The model under review builds one solid part; all positions refer to its coordinate system, in mm. A direction names the side the tool comes from. Coordinates: 2 decimals unless noted, no trailing zeros. Write each loop counter-clockwise with the first axis right and the second up, starting at its lowest first coordinate (ties: lowest second). Pieces come first, ordered by that corner, then holes. Notation, with made-up numbers: (74, 53.25) - (82, 53.25) arc R14 cw to (82, 72.25) - close; hole circle Ø10 at (41.25, 32.25). An arc over 180 degrees is marked (long way). Use one line per item in the form item = value. Start each with the question number.
```python
from build123d import *

# Parameters (mm, degrees)
SKETCH_1_W      = 4.64
SKETCH_1_H      = 2.54
SKETCH_1_W_2    = 0.64
SKETCH_1_H_2    = 0.64
EXTRUDE_1_DEPTH = 6
SKETCH_2_W      = 4.64
SKETCH_2_H      = 2.54
SKETCH_2_R      = 0.45254834
EXTRUDE_2_DEPTH = 3
CHAMFER_1_SIZE  = 0.5


with BuildPart() as part:
    # Эскиз1 → Бобышка-Вытянуть1 (new body)
    with BuildSketch(Plane(origin=(0, 0, 0), x_dir=(1, 0, 0), z_dir=(0, 1, 0))):
        Rectangle(SKETCH_1_W, SKETCH_1_H)
        with Locations((-1.27, 0)):
            Rectangle(SKETCH_1_W_2, SKETCH_1_H_2, mode=Mode.SUBTRACT)
        with Locations((1.27, 0)):
            Rectangle(SKETCH_1_W_2, SKETCH_1_H_2, mode=Mode.SUBTRACT)
    extrude(amount=EXTRUDE_1_DEPTH)

    # Эскиз2 → Бобышка-Вытянуть2 (add)
    with BuildSketch(Plane(origin=(0, 6, 0), x_dir=(1, 0, 0), z_dir=(0, 1, 0))):
        Rectangle(SKETCH_2_W, SKETCH_2_H)
        with Locations((-1.27, 0)):
            Circle(SKETCH_2_R, mode=Mode.SUBTRACT)
        with Locations((1.27, 0)):
            Circle(SKETCH_2_R, mode=Mode.SUBTRACT)
    extrude(amount=EXTRUDE_2_DEPTH)

    # Фаска1
    chamfer_1_edges = [part.edges().sort_by_distance(p)[0] for p in [
        (2.32, 4.5, 1.27),
        (-2.32, 4.5, 1.27),
        (-2.32, 4.5, -1.27),
        (2.32, 4.5, -1.27),
    ]]
    chamfer(chamfer_1_edges, length=CHAMFER_1_SIZE)


solid = part.part
```
1. For faces 4 (the cylindrical face through (-1.722, 7.479, -0.02)), 5 (the flat face through (-2.32, 4, 0)), list the 3-axis set-ups (+Z, -Z, +X, -X, +Y, -Y) from which the entire face can be reached by the end or side of a thin tool; tool diameter is ignored.
2. For L1, parallel to X at y = 5.75, z = -0.25; L2, parallel to X at y = 7.65, z = 0; L3, parallel to Z at x = 1.27, y = 6.8, list the stretches that pass through material, from the lowest coordinate up.
3. The part is to be moulded in two halves that separate along X. For faces 1 (the flat face through (2.32, 4, 0)), 2 (the cylindrical face through (0.911, 7.479, 0.275)), 3 (the flat face through (0, 4, -1.27)), say which applies: released by +X, released by -X, zero draft, split by the parting line, or undercut.
4. Take a section at C-C (z = 0). State the section outline as (x, y) points, plus the area to 3 significant figures.
5. Take a section at B-B (y = 7.5). State the section outline as (x, z) points, plus the area to 4 significant figures.
6. Take a section at A-A (x = 1.27). State the section outline as (y, z) points.
7. Take a section at D-D (y = 4). State the section outline as (x, z) points.
Returned:
q1.face_4 = +Y
q1.face_5 = +Z, -Z, -X, +Y, -Y
q2.L1 = -2.32 to -1.59, -0.95 to 0.95, 1.59 to 2.32
q2.L2 = -2.32 to -1.72, -0.82 to 0.82, 1.72 to 2.32
q2.L3 = -1.27 to -0.45, 0.45 to 1.27
q3.face_1 = released by +X
q3.face_2 = undercut
q3.face_3 = zero draft
q4.outline = (-2.32, 0) - (-1.59, 0) - (-1.59, 6) - (-1.72, 6) - (-1.72, 9) - (-2.32, 9) - close; (-0.95, 0) - (0.95, 0) - (0.95, 6) - (0.82, 6) - (0.82, 9) - (-0.82, 9) - (-0.82, 6) - (-0.95, 6) - close; (1.59, 0) - (2.32, 0) - (2.32, 9) - (1.72, 9) - (1.72, 6) - (1.59, 6) - close
q4.area = 28.6 mm²
q5.outline = (-2.32, -0.77) - (-1.82, -1.27) - (1.82, -1.27) - (2.32, -0.77) - (2.32, 0.77) - (1.82, 1.27) - (-1.82, 1.27) - (-2.32, 0.77) - close; hole circle Ø0.91 at (-1.27, 0); hole circle Ø0.91 at (1.27, 0)
q5.area = 10.00 mm²
q6.outline = (0, -1.27) - (9, -1.27) - (9, -0.45) - (6, -0.45) - (6, -0.32) - (0, -0.32) - close; (0, 0.32) - (6, 0.32) - (6, 0.45) - (9, 0.45) - (9, 1.27) - (0, 1.27) - close
q7.outline = (-2.32, -0.77) - (-1.82, -1.27) - (1.82, -1.27) - (2.32, -0.77) - (2.32, 0.77) - (1.82, 1.27) - (-1.82, 1.27) - (-2.32, 0.77) - close; hole (-1.59, -0.32) - (-0.95, -0.32) - (-0.95, 0.32) - (-1.59, 0.32) - close; hole (0.95, -0.32) - (1.59, -0.32) - (1.59, 0.32) - (0.95, 0.32) - close
